Can you work these out from the model? Positions are in its coordinate system, mm. Face numbers are marked on the shaded views. A direction names the side the tool comes from. Give positions to 0.01 mm unless a question says otherwise; leave off trailing zeros. Order: outer loops, then holes, each group sorted by start corner. A loop starts at its lowest first (then second) coordinate and runs counter-clockwise, first axis right, second up.
Item 1: Which directions (+Z, -Z, +X, -X, +Y, -Y) give clear straight access to the entire face, cutting with the end or side of a thin tool? Please do the marked faces 4 and 5.
Item 2: If I drill on line 1 along Y through (x, z) = (0, -9.5); line 2 along X through (y, z) = (-2, -5.5); line 3 along X through (y, z) = (4.5, -13), over which ranges is the centre line in solid material (lowest first)?
Item 3: I want a section at B-B, the plane x = 0. Write out the boundary of the cut face in (y, z), then the cut area to 3 significant figures.
Item 4: I want a section at D-D, the plane z = 22.5. Write out the boundary of the cut face in (x, y), then the cut area to 3 significant figures.
Item 5: I'm going to push flat-ended pins straight in: pin 1 Ø5 at (x, z) = (3.5, -4.5) entering from -Y; pin 2 Ø6.5 at (x, y) = (5, 4.5) entering from +Z; pin 3 Ø1 at (x, z) = (4.5, -19) entering from -Y; pin 4 Ø1 at (x, z) = (7.5, -17) entering from +Y. Where does each tip first touch, or does it pass through?
Item 6: If we mould it in two halves opening along X, with no side actions, what happens to the marked faces 1, 2 and 3? For each: +X half, -X half, draft (parallel to the pull), parting line (faces both ways), or undercut.
Item 7: I want a section at A-A, the plane z = -8. Write out the boundary of the cut face in (x, y).
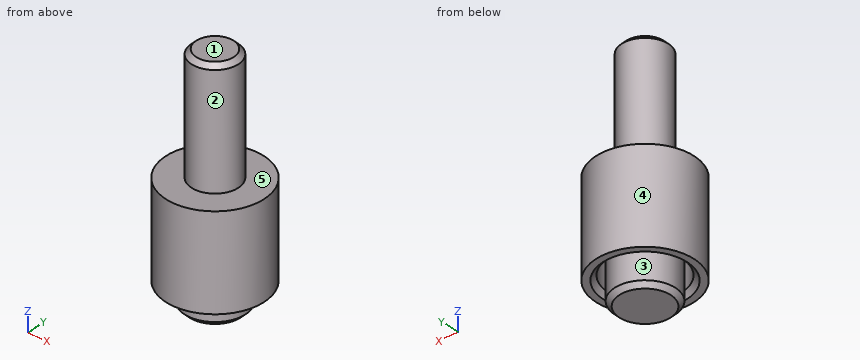
```python
from build123d import *

# Parameters (mm, degrees)
F0_R     = 5
F1_DEPTH = 25
F0_R_2   = 6.5
F2_DEPTH = 25
F0_R_3   = 8
F3_DEPTH = 5
F0_R_4   = 10.5
F4_DEPTH = 20
F5_SIZE  = 1


with BuildPart() as f1:
    # F0 (on Top) → F1 (new body)
    with BuildSketch(Plane.XY):
        Circle(F0_R)
    extrude(amount=F1_DEPTH)

    # F0 (on Top) → F2 (join)
    with BuildSketch(Plane.XY):
        Circle(F0_R_2)
        Circle(F0_R, mode=Mode.SUBTRACT)
        Circle(F0_R)
    extrude(amount=-F2_DEPTH)

    # F0 (on Top) → F3 (join)
    with BuildSketch(Plane.XY):
        Circle(F0_R_3)
        Circle(F0_R_2, mode=Mode.SUBTRACT)
    extrude(amount=-F3_DEPTH)

    # F0 (on Top) → F4 (join)
    with BuildSketch(Plane.XY):
        Circle(F0_R_4)
        Circle(F0_R_3, mode=Mode.SUBTRACT)
    extrude(amount=-F4_DEPTH)

    # F5
    f5_edges = [f1.edges().sort_by_distance(p)[0] for p in [
        (-8, 0, -20),
        (-6.5, 0, -25),
        (-5, 0, 25),
    ]]
    chamfer(f5_edges, length=F5_SIZE)


solid = f1.part
```
Results list:
1. face 4: +Z, -Z
1. face 5: +Z
2. line 1: y = -10.5 to -8, -6.5 to 6.5, 8 to 10.5
2. line 2: x = -10.31 to -7.75, -6.18 to 6.18, 7.75 to 10.31
2. line 3: x = -9.49 to -6.61, -4.69 to 4.69, 6.61 to 9.49
3. outline: (-10.5, -20) - (-9, -20) - (-8, -19) - (-8, -5) - (-6.5, -5) - (-6.5, -24) - (-5.5, -25) - (5.5, -25) - (6.5, -24) - (6.5, -5) - (8, -5) - (8, -19) - (9, -20) - (10.5, -20) - (10.5, 0) - (5, 0) - (5, 24) - (4, 25) - (-4, 25) - (-5, 24) - (-5, 0) - (-10.5, 0) - close
3. area: 687 mm2
4. outline: circle Ø10 at (0, 0)
4. area: 78.5 mm2
5. pin 1: stops at y = -10.45
5. pin 2: stops at z = 25
5. pin 3: stops at y = -9.71
5. pin 4: stops at y = 7.83
6. face 1: draft
6. face 2: parting line
6. face 3: undercut
7. outline: circle Ø21 at (0, 0); circle Ø13 at (0, 0); hole circle Ø16 at (0, 0)
